from build123d import *
from OCP.BRepFilletAPI import BRepFilletAPI_MakeChamfer

# Parameters (mm, degrees)
ESTRUSIONE_ESTRUSIONE1_DEPTH = 40
FORO_PER_VITE_M4_1_D         = 5.4
FORO_PER_VITE_M4_1_DEPTH     = 15
FORO_PER_VITE_M4_1_TIP       = 1.622323671
ESTRUSIONE_ESTRUSIONE2_DEPTH = 4
FORO_PER_VITE_M4_2_D         = 4.5
FORO_PER_VITE_M4_2_DEPTH     = 80
FORO_PER_VITE_M4_2_TIP       = 1.351936393
RACCORDO1_R                  = 10
RACCORDO2_R                  = 30
SMUSSO1_SIZE                 = 2
SMUSSO1_SIZE2                = 1.629150908


with BuildPart() as part:
    # Schizzo1 → Estrusione-Estrusione1 (new body)
    with BuildSketch(Plane.XY):
        with BuildLine():
            Line((-14.657188407, -3.188546376), (-11, -20))
            Line((-11, -20), (11, -20))
            Line((11, -20), (14.657188407, -3.188546376))
            ThreePointArc((14.657188407, -3.188546376), (14.91405086, -1.603460927), (15, 0))
            Line((15, 0), (38.615528128, 0))
            Line((38.615528128, 0), (44.812497155, -132.20000012))
            Line((44.812497155, -132.20000012), (45, -132.20000012))
            Line((45, -132.20000012), (45, -136.20000012))
            Line((45, -136.20000012), (15, -136.20000012))
            Line((15, -136.20000012), (20.446957648, -116.20000012))
            Line((20.446957648, -116.20000012), (17.109407004, -45))
            Line((17.109407004, -45), (8.25243508, -32.058330072))
            ThreePointArc((8.25243508, -32.058330072), (0, -27.706100894), (-8.25243508, -32.058330072))
            Line((-8.25243508, -32.058330072), (-17.109407004, -45))
            Line((-17.109407004, -45), (-20.446957648, -116.20000012))
            Line((-20.446957648, -116.20000012), (-15, -136.20000012))
            Line((-15, -136.20000012), (-45, -136.20000012))
            Line((-45, -136.20000012), (-45, -132.20000012))
            Line((-45, -132.20000012), (-44.812497155, -132.20000012))
            Line((-44.812497155, -132.20000012), (-38.615528128, 0))
            Line((-38.615528128, 0), (-15, 0))
            ThreePointArc((-15, 0), (-14.91405086, -1.603460927), (-14.657188407, -3.188546376))
        make_face()
    extrude(amount=ESTRUSIONE_ESTRUSIONE1_DEPTH)

    # Foro per Vite M4-1
    with Locations(Plane(origin=(0, 0, 0), x_dir=(1, 0, 0), z_dir=(0, 1, 0))):
        with Locations((-28.115528128, -10), (-28.115528128, -30), (28.115528128, -30), (28.115528128, -10)):
            Hole(FORO_PER_VITE_M4_1_D / 2, depth=FORO_PER_VITE_M4_1_DEPTH)
            with Locations((0, 0, -(FORO_PER_VITE_M4_1_DEPTH + FORO_PER_VITE_M4_1_TIP / 2))):  # 118° drill point
                Cone(0, FORO_PER_VITE_M4_1_D / 2, FORO_PER_VITE_M4_1_TIP, mode=Mode.SUBTRACT)

    # Schizzo6 → Estrusione-Estrusione2 (add)
    with BuildSketch(Plane.XZ.offset(136.20000012)):
        Polygon((-45, 40), (-60, 27.5), (-60, 12.5), (-45, 0), align=None)
        Polygon((45, 40), (60, 27.5), (60, 12.5), (45, 0), align=None)
    extrude(amount=-ESTRUSIONE_ESTRUSIONE2_DEPTH)

    # Foro per Vite M4-2
    with Locations(Plane(origin=(0, -132.20000012, 0), x_dir=(1, 0, 0), z_dir=(0, 1, 0))):
        with Locations((-52.5, -20), (52.5, -20)):
            Hole(FORO_PER_VITE_M4_2_D / 2, depth=FORO_PER_VITE_M4_2_DEPTH)
            with Locations((0, 0, -(FORO_PER_VITE_M4_2_DEPTH + FORO_PER_VITE_M4_2_TIP / 2))):  # 118° drill point
                Cone(0, FORO_PER_VITE_M4_2_D / 2, FORO_PER_VITE_M4_2_TIP, mode=Mode.SUBTRACT)

    # Raccordo1
    raccordo1_edges = [part.edges().sort_by_distance(p)[0] for p in [
        (-60, -134.20000012, 12.5),
        (-60, -134.20000012, 27.5),
        (60, -134.20000012, 27.5),
        (60, -134.20000012, 12.5),
    ]]
    fillet(raccordo1_edges, radius=RACCORDO1_R)

    # Raccordo2
    raccordo2_edges = [part.edges().sort_by_distance(p)[0] for p in [
        (-20.446957648, -116.20000012, 20),
        (20.446957648, -116.20000012, 20),
    ]]
    fillet(raccordo2_edges, radius=RACCORDO2_R)

    # Smusso1: one chamfer whose edges measure the first distance from different faces: ONE call of the kernel's chamfer builder (chamfer() names one face for all edges)
    smusso1_edges_1 = [part.edges().sort_by_distance(p)[0] for p in [
        (-18.667449483, -78.237735256, 40),
        (12.680921042, -38.529165036, 40),
        (-12.680921042, -38.529165036, 40),
        (17.102049114, -128.481749861, 0),
        (17.102049114, -128.481749861, 40),
        (-17.102049114, -128.481749861, 0),
        (-17.102049114, -128.481749861, 40),
        (20.078629399, -116.159495492, 0),
        (20.078629399, -116.159495492, 40),
        (-20.078629399, -116.159495492, 0),
        (-20.078629399, -116.159495492, 40),
        (18.667449483, -78.237735256, 40),
        (-18.667449483, -78.237735256, 0),
        (-44.906248578, -132.20000012, 0),
        (-41.714012642, -66.10000006, 0),
        (-14.91405086, -1.603460927, 0),
        (-12.828594204, -11.594273188, 0),
        (0, -20, 0),
        (12.828594204, -11.594273188, 0),
        (14.91405086, -1.603460927, 0),
        (41.714012642, -66.10000006, 0),
        (44.906248578, -132.20000012, 0),
        (18.667449483, -78.237735256, 0),
        (44.906248578, -132.20000012, 40),
        (41.714012642, -66.10000006, 40),
        (14.91405086, -1.603460927, 40),
        (12.828594204, -11.594273188, 40),
        (0, -27.706100894, 40),
        (0, -20, 40),
        (-12.828594204, -11.594273188, 40),
        (-14.91405086, -1.603460927, 40),
        (-41.714012642, -66.10000006, 40),
        (-44.906248578, -132.20000012, 40),
    ]]
    smusso1_edges_2 = [part.edges().sort_by_distance(p)[0] for p in [
        (-15, -136.20000012, 20),
    ]]
    smusso1_side_2 = [part.faces().sort_by_distance(p)[0] for p in [
        (-35.203995695, -136.20000012, 20),
    ]]
    smusso1_edges_3 = [part.edges().sort_by_distance(p)[0] for p in [
        (15, -136.20000012, 20),
    ]]
    smusso1_side_3 = [part.faces().sort_by_distance(p)[0] for p in [
        (17.102049114, -128.481749861, 20),
    ]]
    smusso1 = BRepFilletAPI_MakeChamfer(part.part.solid().wrapped)
    for e in smusso1_edges_1:
        smusso1.Add(SMUSSO1_SIZE, e.wrapped)
    for e in smusso1_edges_2:
        smusso1.Add(SMUSSO1_SIZE, SMUSSO1_SIZE2, e.wrapped, smusso1_side_2[0].wrapped)  # the first distance lies on this face
    for e in smusso1_edges_3:
        smusso1.Add(SMUSSO1_SIZE, SMUSSO1_SIZE2, e.wrapped, smusso1_side_3[0].wrapped)  # the first distance lies on this face
    add(Compound.cast(smusso1.Shape()), mode=Mode.REPLACE)


solid = part.part
Input: part model. Units: mm. Frame: model coordinates. A direction names the side the tool comes from. Round coordinates to 2 decimals unless told otherwise and drop trailing zeros. Write each loop counter-clockwise with the first axis right and the second up, starting at its lowest first coordinate (ties: lowest second). Pieces come first, ordered by that corner, then holes.
1) Contact query for flat-ended pins moving along their axis: P1, Ø2, axis at x = 5, z = 11.5, coming from the -Y side; P2, Ø10, axis at x = -39, z = 14, coming from the +Y side; P3, Ø6, axis at x = 52.5, z = 20, coming from the +Y side; P4, Ø1, axis at x = 46, y = -112.5, coming from the +Z side. Output: stop coordinate, or through.
2) Cut plane A-A (z = 20). Count the separate pieces of the cut face and the enclosed holes in it, then the cut area to 3 significant figures.
3) Cut plane B-B (x = 52.5). Return the cut outline in (y, z), then the cut area to 3 significant figures.
4) Cut plane C-C (y = -84). Return the cut outline in (x, z), then the cut area to 3 significant figures.
5) Draft query along X for faces 1 (the cylindrical face through (-27.764, -7.605, 27.323)), 2 (the cylindrical face through (-59.03, -134.17, 27.11)), 3 (the flat face through (21, -67, 40)). Return one class per face: pulls with the +X half, pulls with the -X half, needs draft (parallel to the pull), parting line crosses it, or undercut.
6) Cut plane D-D (z = 4). Return the cut outline in (x, y), then the cut area to 3 significant figures.
7) Ray query, L1, parallel to X at y = -91, z = 26; L2, parallel to Z at x = -52.5, y = -134.3; L3, parallel to Y at x = 45.5, z = 8. Return the intervals inside material, ascending.
8) Reachability of faces 4 (the flat face through (-13.649, -12.463, 38.986)), 5 (the flat face through (-18.151, -128.383, 38.986)), 6 (the cylindrical face through (0.136, -27.707, 18.734)), 7 (the conical face through (21.079, -116.338, 0.986)), 8 (the flat face through (0, -20, 20)) from +Z, -Z, +X, -X, +Y, -Y: full face, straight path, thin tool, end or side. Return the list, or none.
Geometry says:
1. P1: stops at y = -29.71
1. P2: stops at y = 0
1. P3: stops at y = -132.2
1. P4: passes through
2. separate pieces: 3
2. enclosed holes: 0
2. area: 7,180 mm2
3. outline: (-136.2, 6.25) - (-132.2, 6.25) - (-132.2, 17.75) - (-136.2, 17.75) - close; (-136.2, 22.25) - (-132.2, 22.25) - (-132.2, 33.75) - (-136.2, 33.75) - close
3. area: 92.0 mm2
4. outline: (-42.55, 2) - (-40.55, 0) - (-20.94, 0) - (-18.94, 2) - (-18.94, 38) - (-20.94, 40) - (-40.55, 40) - (-42.55, 38) - close; (18.94, 2) - (20.94, 0) - (40.55, 0) - (42.55, 2) - (42.55, 38) - (40.55, 40) - (20.94, 40) - (18.94, 38) - close
4. area: 1,870 mm2
5. face 1: undercut
5. face 2: pulls with the -X half
5. face 3: needs draft
6. outline: (-49.8, -136.2) - (-17, -136.2) - (-15.43, -134.63) - (-19.2, -120.76) arc R30 cw to (-20.23, -111.48) - (-17.11, -45) - (-8.25, -32.06) arc R10 cw to (8.25, -32.06) - (17.11, -45) - (20.23, -111.48) arc R30 cw to (19.2, -120.76) - (15.53, -134.27) - (16.63, -136.2) - (49.8, -136.2) - (49.8, -132.2) - (44.81, -132.2) - (38.62, 0) - (15, 0) arc R15 cw to (14.66, -3.19) - (11, -20) - (-11, -20) - (-14.66, -3.19) arc R15 cw to (-15, 0) - (-38.62, 0) - (-44.81, -132.2) - (-49.8, -132.2) - close
6. area: 7,140 mm2
7. L1: x = -42.88 to -19.27, 19.27 to 42.88
7. L2: z = 6.25 to 17.75, 22.25 to 33.75
7. L3: y = -136.2 to -132.2
8. face 4: +Z, +Y
8. face 5: +Z
8. face 6: +Z, -Z, -Y
8. face 7: -Z
8. face 8: +Z, -Z, +Y
